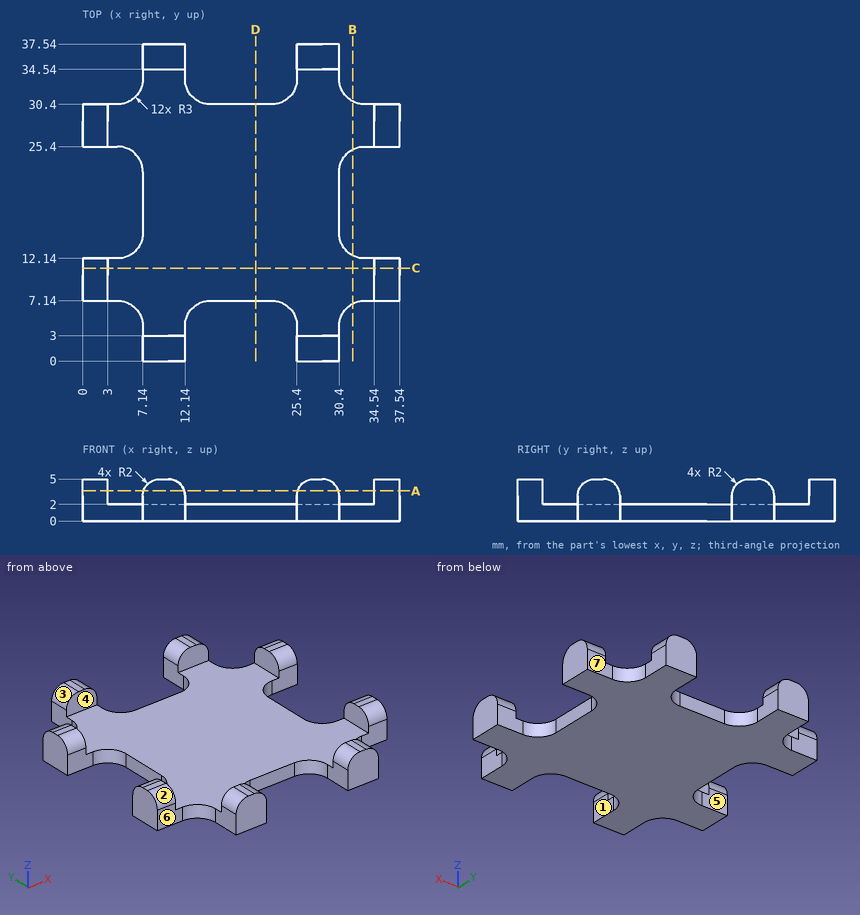
The drawing under review shows one solid part. Ordinate dimensions are in mm from its lowest x, y, z. A direction names the side the tool comes from. Give positions to 0.01 mm unless a question says otherwise; leave off trailing zeros. Order: outer loops, then holes, each group sorted by start corner. A loop starts at its lowest first (then second) coordinate and runs counter-clockwise, first axis right, second up. Notation, with made-up numbers: (75.5, 10) -> (90.5, 10) arc R36 ccw to (90.5, 45) -> close; hole circle Ø2 at (69.25, 33.5). An arc over 180 degrees is marked (long way). Write item = value, one per line. Start each with the question number.
(1) For the marked faces 4, 5, 6 and 7, list the 3-axis set-ups (+Z, -Z, +X, -X, +Y, -Y) from which the entire face can be reached by the end or side of a thin tool; tool diameter is ignored.
(2) We need section A-A on z = 3.6. State how many separate pieces and enclosed holes the cut face has, plus the area to 3 significant figures.
(3) For pin 1 (1 mm diameter, centred on y = 18.5, z = 1, fed in from -X); pin 2 (1.5 mm diameter, centred on y = 21, z = 3.5, fed in from -X); pin 3 (0.9 mm diameter, centred on y = 2, z = 2, fed in from +X); pin 4 (1.5 mm diameter, centred on y = 29, z = 3, fed in from -X), all flat-tipped, find the tip position at first contact; note any pin that passes through.
(4) To check wall thickness, follow line 1 along X through (y, z) = (2.5, 1.6); line 2 along X through (y, z) = (26, 2.7); line 3 along Z through (x, y) = (33, 30). State the ranges of each line that lie inside material, in increasing order.
(5) We need section B-B on x = 32. Write out the cut boundary in (y, z), plus the area to 3 significant figures.
(6) Mouldability with a two-part tool opening along X and no side actions: class the marked faces 1, 2 and 3 as +X half, -X half, draft (parallel to the pull), parting line (faces both ways), or undercut.
(7) We need section D-D on x = 20.5. Write out the cut boundary in (y, z), plus the area to 3 significant figures.
(8) We need section C-C on y = 11. Write out the cut boundary in (x, z), plus the area to 3 significant figures.
Numbers:
q1.face_4 = +Z, +X, -X
q1.face_5 = +Z, -Z, -X
q1.face_6 = +Z, -Z, -X, -Y
q1.face_7 = +Z, -Z, +X, +Y
q2.separate_pieces = 8
q2.enclosed_holes = 0
q2.area = 116 mm^2
q3.pin_1 = 7.14
q3.pin_2 = through
q3.pin_3 = 30.4
q3.pin_4 = 0
q4.line_1 = 7.14 to 12.14, 25.4 to 30.4
q4.line_2 = 0 to 3, 34.54 to 37.54
q4.line_3 = 0 to 2
q5.outline = (6.79, 0) -> (12.49, 0) -> (12.49, 2) -> (6.79, 2) -> close; (25.05, 0) -> (30.75, 0) -> (30.75, 2) -> (25.05, 2) -> close
q5.area = 22.8 mm^2
q6.face_1 = undercut
q6.face_2 = draft
q6.face_3 = -X half
q7.outline = (7.14, 0) -> (30.4, 0) -> (30.4, 2) -> (7.14, 2) -> close
q7.area = 46.5 mm^2
q8.outline = (0, 0) -> (37.54, 0) -> (37.54, 4.81) -> (34.54, 4.81) -> (34.54, 2) -> (3, 2) -> (3, 4.81) -> (0, 4.81) -> close
q8.area = 91.9 mm^2
